Verification items for the finished model (mm, model axes). A direction names the side the tool comes from. Give positions to 0.01 mm unless a question says otherwise; leave off trailing zeros. Write each loop counter-clockwise with the first axis right and the second up, starting at its lowest first coordinate (ties: lowest second). Pieces come first, ordered by that corner, then holes. Notation, with made-up numbers: M 63,10 L 76,10 A23 ccw 76,32 Z; hole C 68.25,54.5 d7. An arc over 180 degrees is marked long. Answer as a JSON object with one key per item and string values.
```python
from build123d import *

# Parameters (mm, degrees)
SKETCH1_W               = 46
SKETCH1_H               = 15
BOSS_EXTRUDE1_DEPTH     = 3
SKETCH3_W               = 2.5
SKETCH3_H               = 15
BOSS_EXTRUDE2_DEPTH     = 20
SKETCH4_W               = 20
SKETCH4_H               = 3
BOSS_EXTRUDE3_DEPTH     = 7
SKETCH5_R               = 2
CUT_EXTRUDE1_DEPTH      = 7
SKETCH7_W               = 9.5
SKETCH7_H               = 15
BOSS_EXTRUDE4_DEPTH     = 10
SKETCH8_R               = 2
CUT_EXTRUDE2_DEPTH      = 10
MIRROR3_COPY_1_SKETCH_W = 9.5
MIRROR3_COPY_1_SKETCH_H = 15
MIRROR3_COPY_1_DEPTH    = 10
MIRROR3_COPY_2_SKETCH_R = 2
MIRROR3_COPY_2_DEPTH    = 10


with BuildPart() as part:
    # Sketch1 → Boss-Extrude1 (new body)
    with BuildSketch(Plane.XY):
        with Locations((23, 7.5)):
            Rectangle(SKETCH1_W, SKETCH1_H)
    extrude(amount=BOSS_EXTRUDE1_DEPTH)

    # Sketch3 → Boss-Extrude2 (add)
    with BuildSketch(Plane.XY.offset(3)):
        with Locations((1.25, 7.5)):
            Rectangle(SKETCH3_W, SKETCH3_H)
    boss_extrude2 = extrude(amount=BOSS_EXTRUDE2_DEPTH)

    # Sketch4 → Boss-Extrude3 (add)
    with BuildSketch(Plane.ZY):
        with Locations((13, 13.5)):
            Rectangle(SKETCH4_W, SKETCH4_H)
    boss_extrude3 = extrude(amount=BOSS_EXTRUDE3_DEPTH)

    # Sketch5 → Cut-Extrude1 (cut)
    with BuildSketch(Plane(origin=(0, 15, 0), x_dir=(1, 0, 0), z_dir=(0, 1, 0))):
        with Locations(Location((-2.25, -18.1, 0), (0, 0, 270))):
            Circle(SKETCH5_R)
        with Locations(Location((-2.25, -7.9, 0), (0, 0, 270))):
            Circle(SKETCH5_R)
    cut_extrude1 = extrude(amount=-CUT_EXTRUDE1_DEPTH, mode=Mode.SUBTRACT)

    # Mirror1: Boss-Extrude2, Boss-Extrude3, Cut-Extrude1 across plane
    add(boss_extrude2.mirror(Plane(origin=(23, 0, 0), x_dir=(0, 0, 1), z_dir=(1, 0, 0))))
    add(boss_extrude3.mirror(Plane(origin=(23, 0, 0), x_dir=(0, 0, 1), z_dir=(1, 0, 0))))
    add(cut_extrude1.mirror(Plane(origin=(23, 0, 0), x_dir=(0, 0, 1), z_dir=(1, 0, 0))), mode=Mode.SUBTRACT)

    # Sketch7 → Boss-Extrude4 (add)
    with BuildSketch(Plane.XY.offset(23)):
        with Locations((-2.25, 7.5)):
            Rectangle(SKETCH7_W, SKETCH7_H)
    boss_extrude4 = extrude(amount=BOSS_EXTRUDE4_DEPTH)

    # Sketch8 → Cut-Extrude2 (cut)
    with BuildSketch(Plane.ZY.offset(7)):
        with Locations((28, 11.25)):
            Circle(SKETCH8_R)
        with Locations((28, 3.75)):
            Circle(SKETCH8_R)
    cut_extrude2 = extrude(amount=-CUT_EXTRUDE2_DEPTH, mode=Mode.SUBTRACT)

    # Mirror2: Boss-Extrude4, Cut-Extrude2 across plane
    add(boss_extrude4.mirror(Plane(origin=(23, 0, 0), x_dir=(0, 0, 1), z_dir=(1, 0, 0))))
    add(cut_extrude2.mirror(Plane(origin=(23, 0, 0), x_dir=(0, 0, 1), z_dir=(1, 0, 0))), mode=Mode.SUBTRACT)

    # Mirror3: Boss-Extrude4, Cut-Extrude2 across plane
    add(boss_extrude4.mirror(Plane.XY.offset(13)))
    add(cut_extrude2.mirror(Plane.XY.offset(13)), mode=Mode.SUBTRACT)

    # Mirror3 copy 1 sketch → Mirror3 copy 1 (add)
    with BuildSketch(Plane(origin=(46, 0, 3), x_dir=(-1, 0, 0), z_dir=(0, 0, -1))):
        with Locations((-2.25, 7.5)):
            Rectangle(MIRROR3_COPY_1_SKETCH_W, MIRROR3_COPY_1_SKETCH_H)
    extrude(amount=MIRROR3_COPY_1_DEPTH)

    # Mirror3 copy 2 sketch → Mirror3 copy 2 (cut)
    with BuildSketch(Plane(origin=(53, 0, 26), x_dir=(0, 0, -1), z_dir=(1, 0, 0))):
        with Locations((28, 11.25)):
            Circle(MIRROR3_COPY_2_SKETCH_R)
        with Locations((28, 3.75)):
            Circle(MIRROR3_COPY_2_SKETCH_R)
    extrude(amount=-MIRROR3_COPY_2_DEPTH, mode=Mode.SUBTRACT)


solid = part.part
```
1) Thickness scan on L1, parallel to X at y = 12.95, z = 7.9; L2, parallel to Y at x = 45.75, z = 28; L3, parallel to X at y = 7.5, z = 23.5. Record the ranges inside material, lowest first.
Completed:
{"L1": "x = -7 to -4.25, -0.25 to 2.5, 43.5 to 46.25, 50.25 to 53", "L2": "y = 0 to 1.75, 5.75 to 9.25, 13.25 to 15", "L3": "x = -7 to 2.5, 43.5 to 53"}
2) Section check A-A on x = -2.25. Record the boundary of the cut face in (y, z), and give its area (3 significant figures).
Completed:
{"outline": "M 0,-7 L 15,-7 L 15,5.9 L 12,5.9 L 12,3 L 0,3 Z; M 0,23 L 12,23 L 12,20.1 L 15,20.1 L 15,33 L 0,33 Z; M 12,9.9 L 15,9.9 L 15,16.1 L 12,16.1 Z; hole C 3.75,-2 d4; hole C 3.75,28 d4; hole C 11.25,-2 d4; hole C 11.25,28 d4", "area": "286 mm2"}
3) Go/stop test with flat-tipped pins: pin 1 (3 mm diameter, centred on x = 10, z = 5, fed in from +Y); pin 2 (1.5 mm diameter, centred on y = 10.5, z = 8.5, fed in from -X); pin 3 (8 mm diameter, centred on y = 6, z = 20.5, fed in from +X); pin 4 (2 mm diameter, centred on y = 9, z = 17.5, fed in from +X). Record where each tip stops, or that it passes through.
Completed:
{"pin 1": "passes through", "pin 2": "stops at x = 0", "pin 3": "stops at x = 53", "pin 4": "stops at x = 46"}
4) Section check D-D on y = 6.75. Record the boundary of the cut face in (x, z), and give its area (3 significant figures).
Completed:
{"outline": "M -7,-7 L 2.5,-7 L 2.5,0 L 43.5,0 L 43.5,-7 L 53,-7 L 53,3 L 46,3 L 46,23 L 53,23 L 53,33 L 43.5,33 L 43.5,3 L 2.5,3 L 2.5,33 L -7,33 L -7,23 L 0,23 L 0,3 L -7,3 Z", "area": "603 mm2"}
5) Release check for a two-part mould opening along X. For faces 1 (the face through (46, 6, 13)), 2 (the face through (-4, 6, 3)), 3 (the face through (23, 8, 0)), 4 (the face through (-7, 12.4, 13.3)) record: pulls with the +X half, pulls with the -X half, needs draft (parallel to the pull), parting line crosses it, or undercut.
Completed:
{"face 1": "pulls with the +X half", "face 2": "needs draft", "face 3": "undercut", "face 4": "pulls with the -X half"}
6) Section check C-C on z = 18.1. Record the boundary of the cut face in (x, y), and give its area (3 significant figures).
Completed:
{"outline": "M -7,12 L -4.25,12 L -4.25,15 L -7,15 Z; M -0.25,12 L 0,12 L 0,0 L 2.5,0 L 2.5,15 L -0.25,15 Z; M 43.5,0 L 46,0 L 46,12 L 46.25,12 L 46.25,15 L 43.5,15 Z; M 50.25,12 L 53,12 L 53,15 L 50.25,15 Z", "area": "93.0 mm2"}
7) Section check B-B on z = 25. Record the boundary of the cut face in (x, y).
Completed:
{"outline": "M -7,0 L 2.5,0 L 2.5,15 L -7,15 Z; M 43.5,0 L 53,0 L 53,15 L 43.5,15 Z"}
8) Access from +Z, -Z, +X, -X, +Y, -Y to the whole of each face (thin tool, end or side, straight path). Record for faces 5 (the face through (-3, 12, 13)), 6 (the face through (2.5, 7, -4)), 7 (the face through (49, 12, 13)), 8 (the face through (23, 8, 3)).
Completed:
{"face 5": "-X, -Y", "face 6": "-Z, +Y, -Y", "face 7": "+X, -Y", "face 8": "+Z, +Y, -Y"}
